from build123d import *

# Parameters (mm, degrees)
SKETCH1_W            = 304.8
SKETCH1_H            = 304.8
BOSS_EXTRUDE1_DEPTH  = 2.9972
SKETCH2_W            = 38.1
SKETCH2_H            = 38.1
CUT_EXTRUDE1_DEPTH   = 2.9972
LPATTERN1_COUNT      = 3
LPATTERN1_PITCH      = 88.9
LPATTERN1_COUNT_DIR2 = 2
LPATTERN1_PITCH_DIR2 = 63.5
CUT_EXTRUDE2_DEPTH   = 2.9972


with BuildPart() as part:
    # Sketch1 → Boss-Extrude1 (new body)
    with BuildSketch(Plane(origin=(0, 0, 0), x_dir=(1, 0, 0), z_dir=(0, 1, 0))):
        Rectangle(SKETCH1_W, SKETCH1_H)
    extrude(amount=BOSS_EXTRUDE1_DEPTH)

    # Sketch2 → Cut-Extrude1 (cut)
    with BuildSketch(Plane(origin=(0, 2.9972, 0), x_dir=(1, 0, 0), z_dir=(0, 1, 0))):
        with Locations((-88.9, 88.9)):
            Rectangle(SKETCH2_W, SKETCH2_H)
    cut_extrude1 = extrude(amount=-CUT_EXTRUDE1_DEPTH, mode=Mode.SUBTRACT)

    # LPattern1: Cut-Extrude1 3 × 2
    with Locations(*[(i * LPATTERN1_PITCH, 0, j * LPATTERN1_PITCH_DIR2) for i in range(LPATTERN1_COUNT) for j in range(LPATTERN1_COUNT_DIR2) if (i, j) != (0, 0)]):
        add(cut_extrude1, mode=Mode.SUBTRACT)

    # Sketch3 → Cut-Extrude2 (cut)
    with BuildSketch(Plane(origin=(0, 2.9972, 0), x_dir=(1, 0, 0), z_dir=(0, 1, 0))):
        Polygon((-69.85, 107.95), (-69.85, 120.65), (12.7, 120.65), (12.7, 107.95), (19.05, 107.95), (19.05, 120.65), (101.6, 120.65), (101.6, 107.95), (107.95, 107.95), (107.95, 120.65), (152.4, 120.65), (152.4, 133.35), (-76.2, 133.35), (-76.2, 107.95), align=None)
        Polygon((-69.85, 6.35), (-69.85, -6.35), (12.7, -6.35), (12.7, 6.35), (19.05, 6.35), (19.05, -6.35), (101.6, -6.35), (101.6, 6.35), (107.95, 6.35), (107.95, -6.35), (152.4, -6.35), (152.4, -19.05), (-76.2, -19.05), (-76.2, 6.35), align=None)
    extrude(amount=-CUT_EXTRUDE2_DEPTH, mode=Mode.SUBTRACT)


solid = part.part
Read the model definition and answer for the solid it produces. Units are mm, in the model's axes. Coordinates: 2 decimals unless noted, no trailing zeros. Order: outer loops, then holes, each group sorted by start corner. A loop starts at its lowest first (then second) coordinate and runs counter-clockwise, first axis right, second up. Notation, with made-up numbers: (40.25, 46.25) - (90.25, 46.25) arc R11 cw to (90.25, 61.25) - close; hole circle Ø2 at (-24, -20.75). An arc over 180 degrees is marked (long way). Use one line per item in the form item = value.
(1) Section B-B, the plane x = -82.5 is taken. Give the vertices of the cut face in (y, z), then the cut area to 3 significant figures.
Computed values:
outline = (0, -152.4) - (3, -152.4) - (3, -107.95) - (0, -107.95) - close; (0, -69.85) - (3, -69.85) - (3, -44.45) - (0, -44.45) - close; (0, -6.35) - (3, -6.35) - (3, 152.4) - (0, 152.4) - close
area = 685 mm²
(2) Section A-A, the plane x = -15 is taken. Give the vertices of the cut face in (y, z), then the cut area to 3 significant figures.
Computed values:
outline = (0, -152.4) - (3, -152.4) - (3, -133.35) - (0, -133.35) - close; (0, -120.65) - (3, -120.65) - (3, -107.95) - (0, -107.95) - close; (0, -69.85) - (3, -69.85) - (3, -44.45) - (0, -44.45) - close; (0, -6.35) - (3, -6.35) - (3, 6.35) - (0, 6.35) - close; (0, 19.05) - (3, 19.05) - (3, 152.4) - (0, 152.4) - close
area = 609 mm²
(3) Straight lines are drawn through the part: L1, parallel to Z at x = -68, y = 1; L2, parallel to X at y = 0.65, z = -77; L3, parallel to Z at x = 6, y = 2.4. For each, find the intervals that lie inside material, in ascending order.
Computed values:
L1 = -152.4 to -133.35, -120.65 to 6.35, 19.05 to 152.4
L2 = -152.4 to -107.95, -69.85 to -19.05, 19.05 to 69.85, 107.95 to 152.4
L3 = -152.4 to -133.35, -120.65 to -107.95, -69.85 to -44.45, -6.35 to 6.35, 19.05 to 152.4
(4) Section C-C, the plane z = -82.5 is taken. Give the vertices of the cut face in (x, y), then the cut area to 3 significant figures.
Computed values:
outline = (-152.4, 0) - (-107.95, 0) - (-107.95, 3) - (-152.4, 3) - close; (-69.85, 0) - (-19.05, 0) - (-19.05, 3) - (-69.85, 3) - close; (19.05, 0) - (69.85, 0) - (69.85, 3) - (19.05, 3) - close; (107.95, 0) - (152.4, 0) - (152.4, 3) - (107.95, 3) - close
area = 571 mm²
